The model under review builds one solid part; all positions refer to its coordinate system, in mm. A direction names the side the tool comes from. Round coordinates to 2 decimals unless told otherwise and drop trailing zeros. Loops run counter-clockwise (first coordinate to the right, second up) from the corner with the lowest first, then second, coordinate; pieces in that order, holes last. Notation, with made-up numbers: (28.25, -18.75) -> (48.25, -18.75) arc R21 ccw to (48.25, 0.25) -> close; hole circle Ø5 at (82, 79.5). An arc over 180 degrees is marked (long way). Use a Markdown table: item, result. Add a question column.
1) Consider section D-D on z = 2. Give the boundary of the cut face in (x, y).
2) Insertion check: pin 1 (23 mm diameter, centred on x = 20, y = 0, fed in from -Z); pin 2 (18 mm diameter, centred on x = 20, y = 0, fed in from +Z); pin 3 (5 mm diameter, centred on y = 12.5, z = -1.5, fed in from -X); pin 4 (1.5 mm diameter, centred on y = 14, z = 7.5, fed in from +X). Each pin has a flat end and moves straight along its axis. Give the tip position at first contact, or say it passes through.
3) Mouldability with a two-part tool opening along Y and no side actions: class faces 4 (the cylindrical face through (2.817, 5.411, -2.788)), 5 (the flat face through (7, -9, 11.05)), 6 (the cylindrical face through (34.995, 0.66, -4.479)) as released by +Y, released by -Y, zero draft, split by the parting line, or undercut.
4) Consider section C-C on z = -4.75. Give the boundary of the cut face in (x, y) (3 decimals), plus the area to 3 significant figures.
5) For faces 1 (the cylindrical face through (34.995, 0.66, 5.349)), 2 (the cylindrical face through (27.944, -6.091, -1.486)), 3 (the flat face through (7, -13, 0)), list the 3-axis set-ups (+Z, -Z, +X, -X, +Y, -Y) from which the entire face can be reached by the end or side of a thin tool; tool diameter is ignored.
6) Wall thickness on probe 1 along Y at (x, z) = (20, -3.85) (3 decimals); probe 2 along Z at (x, y) = (32, -5.5); probe 3 along Y at (x, z) = (20, 2.5): over which ranges is each line inside the solid? List them lowest first.
from build123d import *

# Parameters (mm, degrees)
F2_SIZE = 0.5


with BuildPart() as f1:
    # F0 (on Front) → F1 (revolve)
    with BuildSketch(Plane.XZ):
        Polygon((0, 11.05), (0, 0), (1.985, 0), (1.985, -6), (4.99, -6), (4.99, -3), (9.99, -3), (9.99, 0), (4.99, 0), (4.99, 11.05), align=None)
    revolve(axis=Axis((20, 0, 0.0311555341), (0, 0, -1)))

    # F2
    f2_edges = [f1.edges().sort_by_distance(p)[0] for p in [
        (35.01, 0, 11.05),
        (40, 0, 11.05),
        (40, 0, 0),
        (38.015, 0, -6),
        (30.01, 0, -3),
        (30.01, 0, 0),
    ]]
    chamfer(f2_edges, length=F2_SIZE)


solid = f1.part
Result set:
| question | item | result |
|---|---|---|
| 1 | outline | circle Ø40 at (20, 0); hole circle Ø30.02 at (20, 0) |
| 2 | pin 1 | z = -3 |
| 2 | pin 2 | through |
| 2 | pin 3 | x = 3.3 |
| 2 | pin 4 | x = 34.98 |
| 3 | face 4 | split by the parting line |
| 3 | face 5 | zero draft |
| 3 | face 6 | undercut |
| 4 | outline | circle Ø36.03 at (20, 0); hole circle Ø30.02 at (20, 0) |
| 4 | area | 312 mm2 |
| 5 | face 1 | +Z |
| 5 | face 2 | +Z, -Z |
| 5 | face 3 | -Z |
| 6 | probe 1 | -18.015 to -15.01, 15.01 to 18.015 |
| 6 | probe 2 | -3 to 0 |
| 6 | probe 3 | -20 to -15.01, 15.01 to 20 |
